For this review, take the finished solid that the model builds, in its own axes (mm). Round coordinates to 2 decimals unless told otherwise and drop trailing zeros. Order: outer loops, then holes, each group sorted by start corner. A loop starts at its lowest first (then second) coordinate and runs counter-clockwise, first axis right, second up.
from build123d import *

# Parameters (mm, degrees)
BOSS_EXTRUDE1_DEPTH = 3


with BuildPart() as part:
    # Sketch1 → Boss-Extrude1 (new body)
    with BuildSketch(Plane.XY):
        Polygon((0, 27.15), (0, 32.15), (-3, 32.15), (-3, 35.15), (0, 35.15), (0, 164.85), (-3, 164.85), (-3, 167.85), (0, 167.85), (0, 172.85), (6.5, 172.85), (6.5, 170.425), (9, 170.425), (9, 178.425), (6.5, 178.425), (6.5, 176), (0, 176), (0, 181), (-3, 181), (-3, 184), (0, 184), (0, 200), (139.61, 200), (139.61, 184), (142.61, 184), (142.61, 181), (139.61, 181), (139.61, 176), (133.11, 176), (133.11, 178.425), (130.61, 178.425), (130.61, 170.425), (133.11, 170.425), (133.11, 172.85), (139.61, 172.85), (139.61, 167.85), (142.61, 167.85), (142.61, 164.85), (139.61, 164.85), (139.61, 35.15), (142.61, 35.15), (142.61, 32.15), (139.61, 32.15), (139.61, 27.15), (133.11, 27.15), (133.11, 29.575), (130.61, 29.575), (130.61, 21.575), (133.11, 21.575), (133.11, 24), (139.61, 24), (139.61, 19), (142.61, 19), (142.61, 16), (139.61, 16), (139.61, 0), (118.425, 0), (118.425, -3), (115.425, -3), (115.425, 0), (112.5, 0), (112.5, 6.5), (114.925, 6.5), (114.925, 9), (106.925, 9), (106.925, 6.5), (109.35, 6.5), (109.35, 0), (106.425, 0), (106.425, -3), (103.425, -3), (103.425, 0), (36.185, 0), (36.185, -3), (33.185, -3), (33.185, 0), (30.26, 0), (30.26, 6.5), (32.685, 6.5), (32.685, 9), (24.685, 9), (24.685, 6.5), (27.11, 6.5), (27.11, 0), (24.185, 0), (24.185, -3), (21.185, -3), (21.185, 0), (0, 0), (0, 16), (-3, 16), (-3, 19), (0, 19), (0, 24), (6.5, 24), (6.5, 21.575), (9, 21.575), (9, 29.575), (6.5, 29.575), (6.5, 27.15), align=None)
    extrude(amount=-BOSS_EXTRUDE1_DEPTH)


solid = part.part
(1) Wall thickness on L1, parallel to X at y = 178, z = -1.05; L2, parallel to X at y = 190.5, z = -0.15; L3, parallel to Y at x = 74, z = -0.65: over which ranges is each line inside the solid? List them lowest first.
(2) Add section A-A on y = 114. Give the boundary of the cut face in (x, z).
(3) Clearance check with flat-ended pins moving along their axes: P1, Ø1.5, axis at x = 108.5, z = -1.5, coming from the -Y side; P2, Ø0.9, axis at y = 97, z = -1.5, coming from the -X side; P3, Ø1.5, axis at x = -1, z = -2, coming from the +Y side; P4, Ø4, axis at x = 26, y = 143.5, coming from the +Z side. State where each tip first meets the part, or that it passes through.
Here are the results:
1. L1: x = 0 to 6.5, 9 to 130.61, 133.11 to 139.61
1. L2: x = 0 to 139.61
1. L3: y = 0 to 200
2. outline: (0, -3) - (139.61, -3) - (139.61, 0) - (0, 0) - close
3. P1: stops at y = 0
3. P2: stops at x = 0
3. P3: stops at y = 184
3. P4: stops at z = 0
